from build123d import *

# Parameters (mm, degrees)
SKETCH_1_W               = 110
SKETCH_1_H               = 50
EXTRUDE_1_DEPTH          = 60
SKETCH_2_W               = 75
SKETCH_2_H               = 30
CUT_EXTRUDE_1_DEPTH      = 135.907375632
CUT_EXTRUDE_2_DEPTH      = 135.907375632
CUT_EXTRUDE_2_DEPTH_BACK = 135.907375632
CUT_EXTRUDE_3_DEPTH      = 123.983738762
CUT_EXTRUDE_3_DEPTH_BACK = 123.983738762


with BuildPart() as part:
    # 스케치1 → 보스-돌출1 (new body)
    with BuildSketch(Plane(origin=(0, 0, 0), x_dir=(1, 0, 0), z_dir=(0, 1, 0))):
        with Locations((55, 25)):
            Rectangle(SKETCH_1_W, SKETCH_1_H)
    extrude(amount=EXTRUDE_1_DEPTH)

    # 스케치2 → 컷-돌출1 (cut, through all)
    with BuildSketch(Plane(origin=(0, 60, 0), x_dir=(1, 0, 0), z_dir=(0, 1, 0))):
        with Locations((52.5, 15)):
            Rectangle(SKETCH_2_W, SKETCH_2_H)
    extrude(amount=-CUT_EXTRUDE_1_DEPTH, mode=Mode.SUBTRACT)

    # 스케치4 → 컷-돌출2 (cut, two sides: drawn at the far end of the back side and taken through both)
    with BuildSketch(Plane.XY.offset(-CUT_EXTRUDE_2_DEPTH_BACK)):
        Polygon((-171.932939983, 181.104537133), (40, 60), (110, 20), (321.932939983, -101.104537133), (564.14201425, 322.761342833), (70.276134283, 604.9704171), align=None)
    extrude(amount=CUT_EXTRUDE_2_DEPTH + CUT_EXTRUDE_2_DEPTH_BACK, mode=Mode.SUBTRACT)

    # 스케치5 → 컷-돌출3 (cut, two sides: drawn at the far end of the back side and taken through both)
    with BuildSketch(Plane(origin=(15, 0, 0), x_dir=(0, 0, -1), z_dir=(1, 0, 0)).offset(-CUT_EXTRUDE_3_DEPTH_BACK)):
        Polygon((155.435378317, 127.717689158), (20, 60), (0, 50), (-135.435378317, -17.717689158), (-270.870756633, 253.153067475), (20, 398.588445792), align=None)
    extrude(amount=CUT_EXTRUDE_3_DEPTH + CUT_EXTRUDE_3_DEPTH_BACK, mode=Mode.SUBTRACT)


solid = part.part
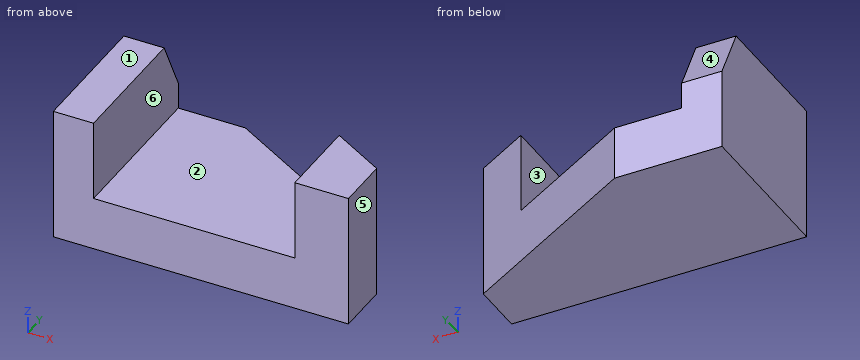
Input: part model. Units: mm. Frame: model coordinates. Face numbers are marked on the shaded views. A direction names the side the tool comes from. Give positions to 0.01 mm unless a question says otherwise; leave off trailing zeros. Loops run counter-clockwise (first coordinate to the right, second up) from the corner with the lowest first, then second, coordinate; pieces in that order, holes last. Notation, with made-up numbers: (78, 25.5) -> (134, 25.5) arc R26 cw to (134, 60.5) -> close; hole circle Ø7 at (-31.5, 77.25). An arc over 180 degrees is marked (long way). Answer as a JSON object with one key per item and string values. Group by question number.
Item 1: Cut plane A-A, the plane z = -4. Return the cut outline in (x, y).
Item 2: Cut plane D-D, the plane y = 17.5. Return the cut outline in (x, z), and give its area (3 significant figures).
Item 3: Reachability of the marked faces 1 and 2 from +Z, -Z, +X, -X, +Y, -Y: full face, straight path, thin tool, end or side. Return the list, or none.
Item 4: Pull-direction query (X, two-part tool) for the marked faces 3, 4, 5 and 6; classes: released by +X, released by -X, zero draft, split by the parting line, or undercut.
Item 5: Pin query (flat end, axial travel): P1, Ø2, axis at x = 85.5, y = 33.5, coming from the +Z side; P2, Ø5, axis at x = 56, z = -27, coming from the +Y side. Return the tip coordinate at first contact, or that it passes through.
Item 6: Line query: probe 1 along X at (y, z) = (9, -26); probe 2 along Z at (x, y) = (61, 42.5); probe 3 along X at (y, z) = (49.5, -27). Output: solid intervals per line, ascending.
Item 7: Cut plane C-C, the plane z = -18.5. Return the cut outline in (x, y).
Item 8: Cut plane B-B, the plane y = 28. Return the cut outline in (x, z).
Checks:
{
 "1": {"outline": "(0, 0) -> (15, 0) -> (15, 52) -> (0, 52) -> close; (90, 0) -> (110, 0) -> (110, 20) -> (90, 31.43) -> close"},
 "2": {"outline": "(0, -50) -> (110, -50) -> (110, 0) -> (90, 0) -> (90, -30) -> (15, -30) -> (15, 0) -> (0, 0) -> close", "area": "3,250 mm²"},
 "3": {"face 1": "+Z, +X, -X, +Y, -Y", "face 2": "+Z, +Y, -Y"},
 "4": {"face 3": "undercut", "face 4": "zero draft", "face 5": "released by +X", "face 6": "undercut"},
 "5": {"P1": "stops at z = -30", "P2": "passes through"},
 "6": {"probe 1": "x = 0 to 15, 90 to 110", "probe 2": "z = -50 to -30", "probe 3": "x = 0 to 15"},
 "7": {"outline": "(0, 0) -> (15, 0) -> (15, 59.25) -> (0, 59.25) -> close; (90, 0) -> (110, 0) -> (110, 20) -> (90, 31.43) -> close"},
 "8": {"outline": "(0, -50) -> (96, -50) -> (96, 0) -> (90, 0) -> (90, -30) -> (15, -30) -> (15, 0) -> (0, 0) -> close"}
}
